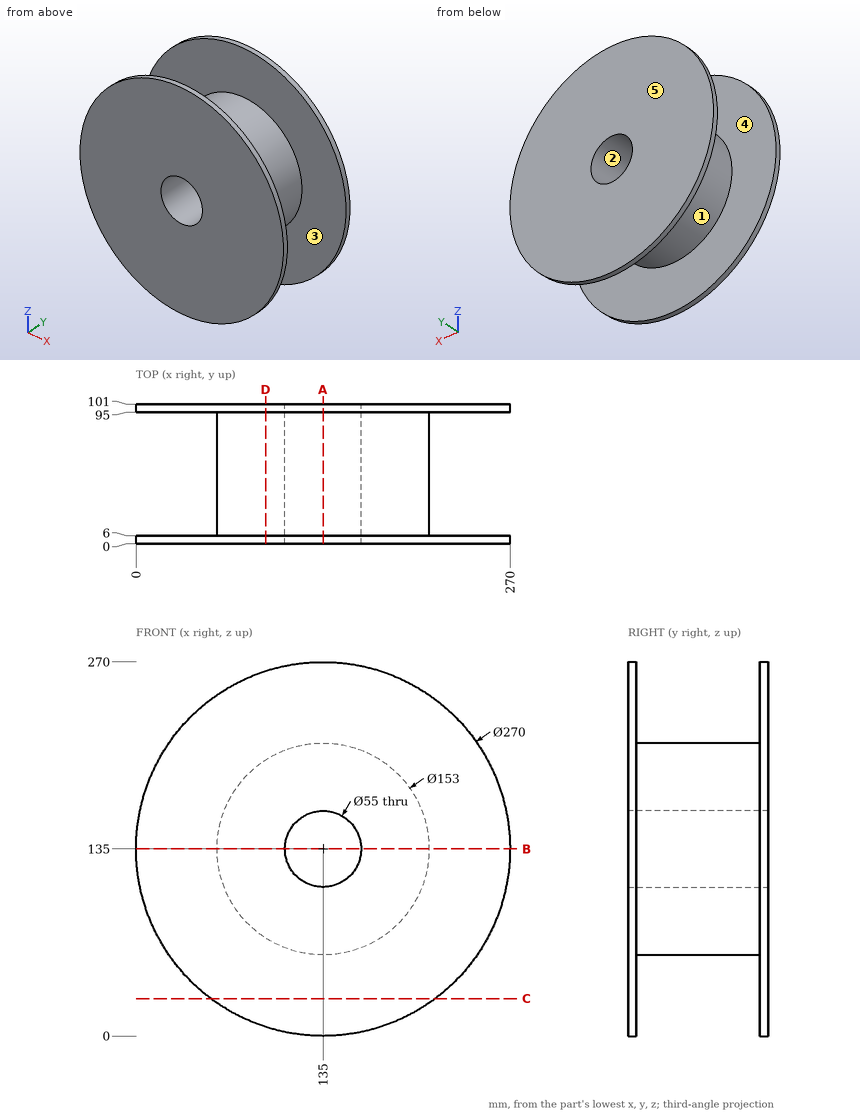
Check sheet for the drawn part. Datum: minimum x, y, z corner. Units: mm. A direction names the side the tool comes from. Coordinates: 2 decimals unless noted, no trailing zeros. Write each loop counter-clockwise with the first axis right and the second up, starting at its lowest first coordinate (ties: lowest second). Pieces come first, ordered by that corner, then holes. Notation, with made-up numbers: (76, 74) - (113, 74) arc R9 cw to (113, 87) - close; hole circle Ø6 at (-14, -3.5). An arc over 180 degrees is marked (long way). Answer as a JSON object with one key per item and string values.
(1) Cross-section at A-A on x = 135. Record the cut outline in (y, z).
Report:
{"outline": "(0, 0) - (6, 0) - (6, 58.5) - (95, 58.5) - (95, 0) - (101, 0) - (101, 107.5) - (0, 107.5) - close; (0, 162.5) - (101, 162.5) - (101, 270) - (95, 270) - (95, 211.5) - (6, 211.5) - (6, 270) - (0, 270) - close"}
(2) Cross-section at D-D on x = 93.5. Record the cut outline in (y, z), plus the area to 3 significant figures.
Report:
{"outline": "(0, 6.54) - (6, 6.54) - (6, 70.73) - (95, 70.73) - (95, 6.54) - (101, 6.54) - (101, 263.46) - (95, 263.46) - (95, 199.27) - (6, 199.27) - (6, 263.46) - (0, 263.46) - close", "area": "14,500 mm^2"}
(3) Cross-section at B-B on z = 135. Record the cut outline in (x, y), plus the area to 3 significant figures.
Report:
{"outline": "(0, 0) - (107.5, 0) - (107.5, 101) - (0, 101) - (0, 95) - (58.5, 95) - (58.5, 6) - (0, 6) - close; (162.5, 0) - (270, 0) - (270, 6) - (211.5, 6) - (211.5, 95) - (270, 95) - (270, 101) - (162.5, 101) - close", "area": "11,300 mm^2"}
(4) Gauge pin test, flat ends, axial feed: pin 1 Ø1.5 at (y, z) = (25.5, 170.5) entering from +X; pin 2 Ø4 at (y, z) = (27, 168.5) entering from -X; pin 3 Ø2 at (y, z) = (59, 68) entering from +X. Record the tip position at first contact, or that the pin passes through.
Report:
{"pin 1": "x = 203.15", "pin 2": "x = 65.29", "pin 3": "x = 173.68"}
(5) Tool access check on the marked faces 4 and 5. Record the directions out of +Z, -Z, +X, -X, +Y, -Y that give a thin tool (end or side, any length) a straight path to the whole face; none if there is none.
Report:
{"face 4": "none", "face 5": "+Z, -Z, +X, -X, +Y"}
(6) Cross-section at C-C on z = 27. Record the cut outline in (x, y), plus the area to 3 significant figures.
Report:
{"outline": "(54, 0) - (216, 0) - (216, 6) - (54, 6) - close; (54, 95) - (216, 95) - (216, 101) - (54, 101) - close", "area": "1,940 mm^2"}
(7) Thickness scan on line 1 along Y through (x, z) = (180, 26); line 2 along Z through (x, y) = (136.5, 73); line 3 along X through (y, z) = (66.5, 135). Record the ranges inside material, lowest first.
Report:
{"line 1": "0 to 6, 95 to 101", "line 2": "58.51 to 107.54, 162.46 to 211.49", "line 3": "58.5 to 107.5, 162.5 to 211.5"}
(8) Mould release check, pull along Z, two halves, no side actions. Record for the marked faces 1, 2 and 3: pulls with the +Z half, pulls with the -Z half, needs draft (parallel to the pull), parting line crosses it, or undercut.
Report:
{"face 1": "parting line crosses it", "face 2": "undercut", "face 3": "needs draft"}
